from build123d import *

# Parameters (mm, degrees)
CYLINDER013_R     = 1.65
CYLINDER013_DEPTH = 10
CYLINDER012_R     = 25
CYLINDER012_DEPTH = 10
CYLINDER004_R     = 1.65
CYLINDER004_DEPTH = 10
CYLINDER005_R     = 1.65
CYLINDER005_DEPTH = 10
CYLINDER006_R     = 1.65
CYLINDER006_DEPTH = 10
CYLINDER007_R     = 1.65
CYLINDER007_DEPTH = 10
CYLINDER001_R     = 9
CYLINDER001_DEPTH = 100
CYLINDER002_R     = 9
CYLINDER002_DEPTH = 100
CYLINDER003_R     = 9
CYLINDER003_DEPTH = 100
CYLINDER_R        = 9
CYLINDER_DEPTH    = 100
BOX_W             = 155
BOX_H             = 105
BOX_DEPTH         = 5
CYLINDER009_R     = 25
CYLINDER009_DEPTH = 10
CYLINDER008_R     = 30
CYLINDER008_DEPTH = 5


with BuildPart() as zylinder013:
    # Cylinder013 → Cylinder013 (new body)
    with BuildSketch(Plane(origin=(47.5, 25, 7.5), x_dir=(1, 0, 0), z_dir=(0, -1, 0))):
        Circle(CYLINDER013_R)
    extrude(amount=CYLINDER013_DEPTH)


with BuildPart() as zylinder012:
    # Cylinder012 → Cylinder012 (new body)
    with BuildSketch(Plane(origin=(47.5, 47.5, 0), x_dir=(1, 0, 0), z_dir=(0, 0, 1))):
        Circle(CYLINDER012_R)
    extrude(amount=CYLINDER012_DEPTH)


with BuildPart() as zylinder004:
    # Cylinder004 → Cylinder004 (new body)
    with BuildSketch(Plane(origin=(10, 5, 2.5), x_dir=(1, 0, 0), z_dir=(0, -1, 0))):
        Circle(CYLINDER004_R)
    extrude(amount=CYLINDER004_DEPTH)


with BuildPart() as zylinder005:
    # Cylinder005 → Cylinder005 (new body)
    with BuildSketch(Plane(origin=(10, 100, 2.5), x_dir=(1, 0, 0), z_dir=(0, -1, 0))):
        Circle(CYLINDER005_R)
    extrude(amount=CYLINDER005_DEPTH)


with BuildPart() as zylinder006:
    # Cylinder006 → Cylinder006 (new body)
    with BuildSketch(Plane(origin=(135, 5, 2.5), x_dir=(1, 0, 0), z_dir=(0, -1, 0))):
        Circle(CYLINDER006_R)
    extrude(amount=CYLINDER006_DEPTH)


with BuildPart() as compound001:
    # Cylinder007 → Cylinder007 (new body)
    with BuildSketch(Plane(origin=(135, 100, 2.5), x_dir=(1, 0, 0), z_dir=(0, -1, 0))):
        Circle(CYLINDER007_R)
    extrude(amount=CYLINDER007_DEPTH)

    # Compound001: union Zylinder004, Zylinder005, Zylinder006
    add(zylinder004.part)
    add(zylinder005.part)
    add(zylinder006.part)


with BuildPart() as zylinder001:
    # Cylinder001 → Cylinder001 (new body)
    with BuildSketch(Plane(origin=(135, 85, -10), x_dir=(1, 0, 0), z_dir=(0, 0, 1))):
        Circle(CYLINDER001_R)
    extrude(amount=CYLINDER001_DEPTH)


with BuildPart() as zylinder002:
    # Cylinder002 → Cylinder002 (new body)
    with BuildSketch(Plane(origin=(10, 85, -10), x_dir=(1, 0, 0), z_dir=(0, 0, 1))):
        Circle(CYLINDER002_R)
    extrude(amount=CYLINDER002_DEPTH)


with BuildPart() as zylinder003:
    # Cylinder003 → Cylinder003 (new body)
    with BuildSketch(Plane(origin=(135, 10, -10), x_dir=(1, 0, 0), z_dir=(0, 0, 1))):
        Circle(CYLINDER003_R)
    extrude(amount=CYLINDER003_DEPTH)


with BuildPart() as posts1:
    # Cylinder → Cylinder (new body)
    with BuildSketch(Plane(origin=(10, 10, -10), x_dir=(1, 0, 0), z_dir=(0, 0, 1))):
        Circle(CYLINDER_R)
    extrude(amount=CYLINDER_DEPTH)

    # Compound: union Zylinder001, Zylinder002, Zylinder003
    add(zylinder001.part)
    add(zylinder002.part)
    add(zylinder003.part)


with BuildPart() as cut004:
    # Box → Box (new body)
    with BuildSketch(Plane(origin=(-5, -5, 0), x_dir=(1, 0, 0), z_dir=(0, 0, 1))):
        with Locations((77.5, 52.5)):
            Rectangle(BOX_W, BOX_H)
    extrude(amount=BOX_DEPTH)

    # Cut: cut Posts1
    add(posts1.part, mode=Mode.SUBTRACT)

    # Cut001: cut Compound001
    add(compound001.part, mode=Mode.SUBTRACT)

    # Cut004: cut Zylinder012
    add(zylinder012.part, mode=Mode.SUBTRACT)


with BuildPart() as zylinder009:
    # Cylinder009 → Cylinder009 (new body)
    with BuildSketch(Plane(origin=(47.5, 47.5, 0), x_dir=(1, 0, 0), z_dir=(0, 0, 1))):
        Circle(CYLINDER009_R)
    extrude(amount=CYLINDER009_DEPTH)


with BuildPart() as plate:
    # Cylinder008 → Cylinder008 (new body)
    with BuildSketch(Plane(origin=(47.5, 47.5, 5), x_dir=(1, 0, 0), z_dir=(0, 0, 1))):
        Circle(CYLINDER008_R)
    extrude(amount=CYLINDER008_DEPTH)

    # Cut002: cut Zylinder009
    add(zylinder009.part, mode=Mode.SUBTRACT)

    # Fusion: union Cut004
    add(cut004.part)

    # Cut005: cut Zylinder013
    add(zylinder013.part, mode=Mode.SUBTRACT)


solid = plate.part
Verification items for the finished model (mm, model axes). A direction names the side the tool comes from. Coordinates: 2 decimals unless noted, no trailing zeros. Write each loop counter-clockwise with the first axis right and the second up, starting at its lowest first coordinate (ties: lowest second). Pieces come first, ordered by that corner, then holes. Notation, with made-up numbers: (-27.5, 27) - (25.5, 27) arc R26 cw to (25.5, 42) - close; hole circle Ø11 at (35, 42). An arc over 180 degrees is marked (long way). Answer as a JSON object with one key per item and string values.
(1) Cross-section at B-B on x = 135. Record the cut outline in (y, z).
Report:
{"outline": "(-5, 0) - (1, 0) - (1, 0.85) - (-5, 0.85) - close; (-5, 4.15) - (1, 4.15) - (1, 5) - (-5, 5) - close; (19, 0) - (76, 0) - (76, 5) - (19, 5) - close; (94, 0) - (100, 0) - (100, 0.85) - (94, 0.85) - close; (94, 4.15) - (100, 4.15) - (100, 5) - (94, 5) - close"}
(2) Gauge pin test, flat ends, axial feed: pin 1 Ø2.5 at (x, z) = (135, 2.5) entering from +Y; pin 2 Ø2.5 at (x, z) = (10, 2.5) entering from -Y; pin 3 Ø6 at (x, y) = (97.5, 84.5) entering from +Z. Record the tip position at first contact, or that the pin passes through.
Report:
{"pin 1": "y = 76.09", "pin 2": "y = 18.91", "pin 3": "z = 5"}
(3) Cross-section at A-A on y = 85. Record the cut outline in (x, z), plus the area to 3 significant figures.
Report:
{"outline": "(-5, 0) - (1, 0) - (1, 5) - (-5, 5) - close; (19, 0) - (126, 0) - (126, 5) - (19, 5) - close; (144, 0) - (150, 0) - (150, 5) - (144, 5) - close", "area": "595 mm^2"}
(4) Mould release check, pull along Y, two halves, no side actions. Record for faces 1 (the flat face through (89, 48, 5)), 2 (the cylindrical face through (27.66, 32.29, 4.93)), 3 (the flat face through (71, 100, 2)), 4 (the cylindrical face through (139.153, 77.015, 2.465)): pulls with the +Y half, pulls with the -Y half, needs draft (parallel to the pull), parting line crosses it, or undercut.
Report:
{"face 1": "needs draft", "face 2": "undercut", "face 3": "pulls with the +Y half", "face 4": "undercut"}
(5) Cross-section at C-C on z = 2.5. Record the cut outline in (x, y), plus the area to 3 significant figures.
Report:
{"outline": "(-5, -5) - (8.35, -5) - (8.35, 1.15) arc R9 cw (long way) to (11.65, 1.15) - (11.65, -5) - (133.35, -5) - (133.35, 1.15) arc R9 cw (long way) to (136.65, 1.15) - (136.65, -5) - (150, -5) - (150, 100) - (136.65, 100) - (136.65, 93.85) arc R9 cw (long way) to (133.35, 93.85) - (133.35, 100) - (11.65, 100) - (11.65, 93.85) arc R9 cw (long way) to (8.35, 93.85) - (8.35, 100) - (-5, 100) - close; hole circle Ø50 at (47.5, 47.5)", "area": "13,200 mm^2"}
(6) Tool access check on faces 5 (the flat face through (150, 47, 2)), 6 (the cylindrical face through (40.997, 18.213, 7.465)), 7 (the cylindrical face through (136.574, 96.965, 2.996)), 8 (the cylindrical face through (10.89, -1.88, 3.89)), 9 (the cylindrical face through (143.314, 6.553, 2.465)). Record the directions out of +Z, -Z, +X, -X, +Y, -Y that give a thin tool (end or side, any length) a straight path to the whole face; none if there is none.
Report:
{"face 5": "+Z, -Z, +X, +Y, -Y", "face 6": "+Z", "face 7": "+Y", "face 8": "-Y", "face 9": "+Z, -Z"}
(7) Thickness scan on line 1 along X through (y, z) = (85, 3); line 2 along X through (y, z) = (-2, 2.5); line 3 along Z through (x, y) = (10, 97.5). Record the ranges inside material, lowest first.
Report:
{"line 1": "-5 to 1, 19 to 126, 144 to 150", "line 2": "-5 to 8.35, 11.65 to 133.35, 136.65 to 150", "line 3": "0 to 0.85, 4.15 to 5"}
(8) Cross-section at D-D on y = 47.5. Record the cut outline in (x, z), plus the area to 3 significant figures.
Report:
{"outline": "(-5, 0) - (22.5, 0) - (22.5, 10) - (17.5, 10) - (17.5, 5) - (-5, 5) - close; (72.5, 0) - (150, 0) - (150, 5) - (77.5, 5) - (77.5, 10) - (72.5, 10) - close", "area": "575 mm^2"}
